Could you check a few things on this drawing? It's one solid part, dimensions in mm from its lowest x, y, z. A direction names the side the tool comes from. Round coordinates to 2 decimals unless told otherwise and drop trailing zeros. Write each loop counter-clockwise with the first axis right and the second up, starting at its lowest first coordinate (ties: lowest second). Pieces come first, ordered by that corner, then holes. Notation, with made-up numbers: (-1, -37.75) -> (42, -37.75) arc R31 ccw to (42, -4.75) -> close; hole circle Ø8 at (-26.75, 79). An arc over 180 degrees is marked (long way). Answer in a Markdown table with one row per item.
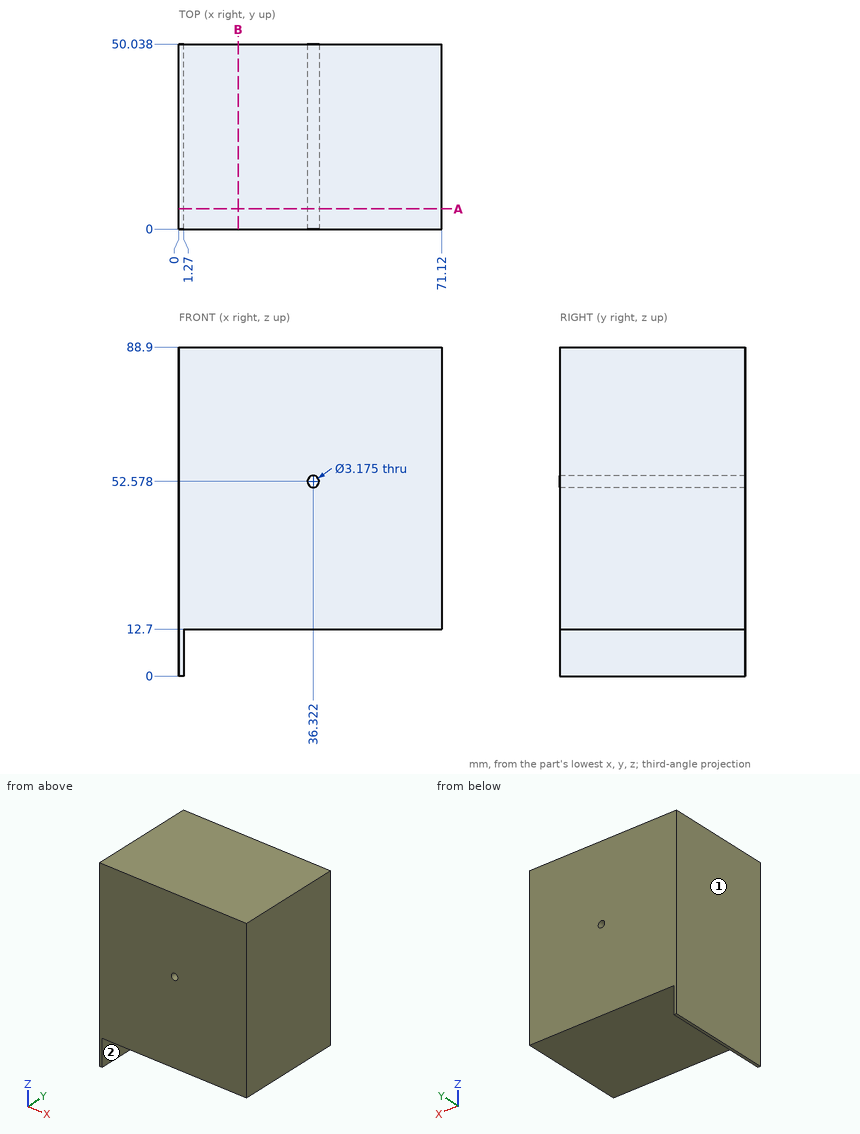
1) For pin 1 (12 mm diameter, centred on x = 8, y = 23, fed in from -Z); pin 2 (8 mm diameter, centred on x = 29.5, z = 76, fed in from -Y); pin 3 (6.5 mm diameter, centred on y = 19.5, z = 8.5, fed in from +X), each with a flat end and sliding along its axis, tell me the tip position at first contact or that it passes through.
Response:
| item | result |
|---|---|
| pin 1 | stops at z = 12.7 |
| pin 2 | stops at y = 0 |
| pin 3 | stops at x = 1.27 |
2) I need wall thicknesses on line 1 (Z direction, x = 19, y = 46); line 2 (X direction, y = 18.5, z = 8). Which ranges of each line are inside material? Lowest first, please. Write a range as [from, to].
Response:
| item | result |
|---|---|
| line 1 | z = [12.7, 88.9] |
| line 2 | x = [0, 1.27] |
3) I want a section at A-A, the plane y = 5.5. List the corners of the cut face in (x, z) for me (1 decimal).
Response:
| item | result |
|---|---|
| outline | (0, 0) -> (1.3, 0) -> (1.3, 12.7) -> (71.1, 12.7) -> (71.1, 88.9) -> (0, 88.9) -> close; hole circle Ø3.2 at (36.3, 52.6) |
4) Which directions (+Z, -Z, +X, -X, +Y, -Y) give clear straight access to the entire face, cutting with the end or side of a thin tool? Please do the marked faces 1 and 2.
Response:
| item | result |
|---|---|
| face 1 | +Z, -Z, -X, +Y, -Y |
| face 2 | -Z, +X, +Y, -Y |
5) I want a section at B-B, the plane x = 16. List the corners of the cut face in (y, z) for me, and give its area (3 significant figures).
Response:
| item | result |
|---|---|
| outline | (0, 12.7) -> (50.04, 12.7) -> (50.04, 88.9) -> (0, 88.9) -> close |
| area | 3,810 mm^2 |
